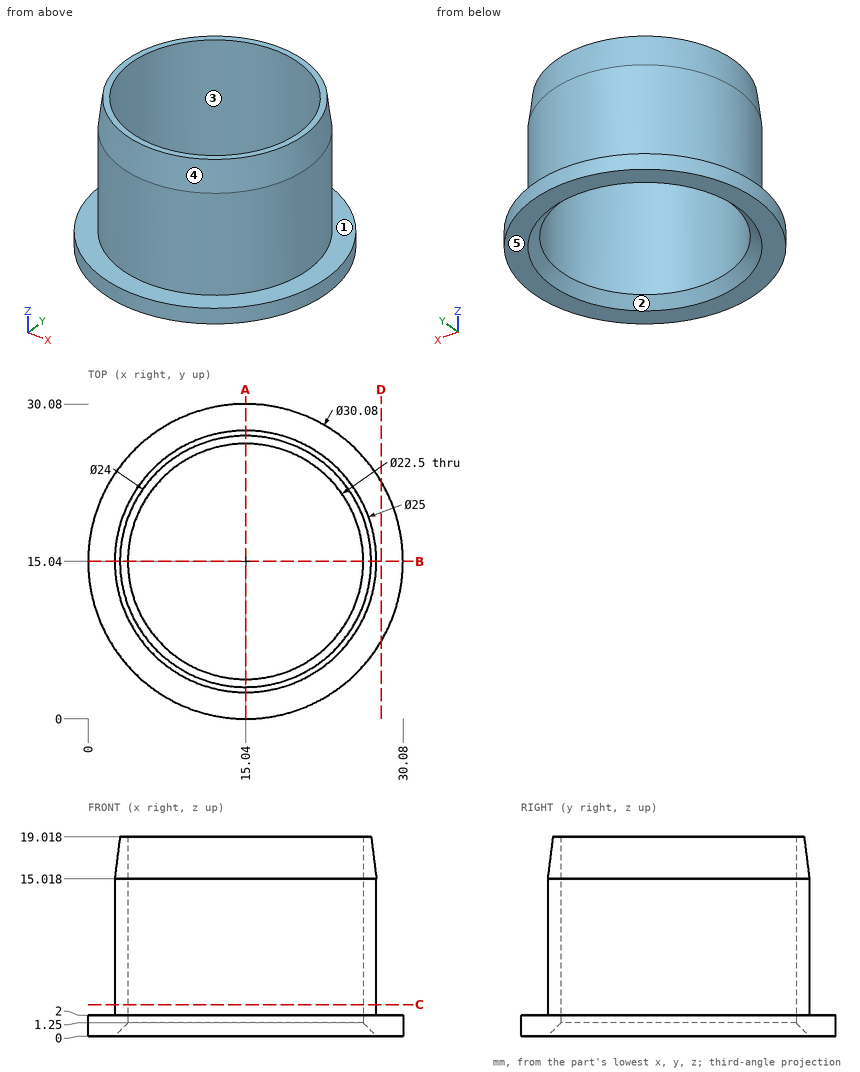
Could you check a few things on this drawing? It's one solid part, dimensions in mm from its lowest x, y, z. A direction names the side the tool comes from. Coordinates: 2 decimals unless noted, no trailing zeros. Order: outer loops, then holes, each group sorted by start corner. A loop starts at its lowest first (then second) coordinate and runs counter-clockwise, first axis right, second up.
1. If we section it at C-C (z = 3): Please give me the cut outline in (x, y).
2. I need wall thicknesses on line 1 (Y direction, x = 15.04, z = 10.75); line 2 (Z direction, x = 18, y = 27.5); line 3 (Y direction, x = 8, z = 6). Which ranges of each line are inside material? Lowest first, please.
3. Thinking about a two-plate mould opening in Y: for the marked faces 3, 4 and 5, which applies, +Y half, -Y half, draft (parallel to the pull), parting line (faces both ways), or undercut?
4. If we section it at A-A (x = 15.04): Please give me the cut outline in (y, z).
5. I'm going to push flat-ended pins straight in: pin 1 (3 mm diameter, centred on x = 16.5, z = 17, fed in from +Y); pin 2 (8 mm diameter, centred on y = 6.5, z = 13, fed in from -X); pin 3 (6 mm diameter, centred on x = 20, z = 2, fed in from +Y). Where does each tip first touch, or does it pass through?
6. For the marked faces 1 and 2, which set-ups out of +Z, -Z, +X, -X, +Y, -Y let a thin tool reach every point of the face, with its end or its side?
7. If we section it at D-D (x = 28): Please give me the cut outline in (y, z).
Entries:
1. outline: circle Ø25 at (15.04, 15.04); hole circle Ø22.5 at (15.04, 15.04)
2. line 1: y = 2.54 to 3.79, 26.29 to 27.54
2. line 2: z = 0 to 2
2. line 3: y = 4.71 to 6.26, 23.82 to 25.37
3. face 3: undercut
3. face 4: parting line
3. face 5: draft
4. outline: (0, 0) - (2.54, 0) - (3.79, 1.25) - (3.79, 19.02) - (3.04, 19.02) - (2.54, 15.02) - (2.54, 2) - (0, 2) - close; (26.29, 1.25) - (27.54, 0) - (30.08, 0) - (30.08, 2) - (27.54, 2) - (27.54, 15.02) - (27.04, 19.02) - (26.29, 19.02) - close
5. pin 1: stops at y = 27.43
5. pin 2: stops at x = 3.39
5. pin 3: stops at y = 29.95
6. face 1: +Z
6. face 2: -Z
7. outline: (7.41, 0) - (22.67, 0) - (22.67, 2) - (7.41, 2) - close
